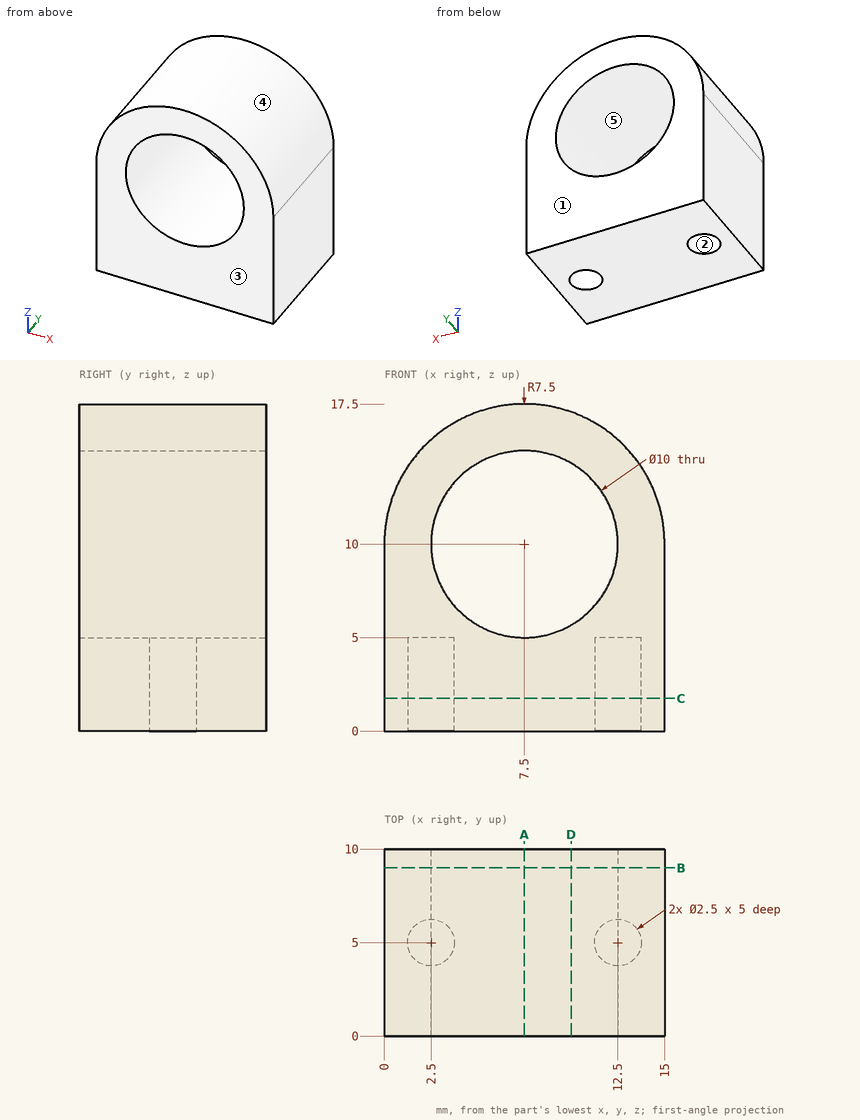
Could you check a few things on this drawing? It's one solid part, dimensions in mm from its lowest x, y, z. A direction names the side the tool comes from. Coordinates: 2 decimals unless noted, no trailing zeros. Loops run counter-clockwise (first coordinate to the right, second up) from the corner with the lowest first, then second, coordinate; pieces in that order, holes last. Notation, with made-up numbers: (4.25, -33) - (31.25, -33) arc R17 ccw to (31.25, -24) - close; hole circle Ø9 at (70.5, 68.25). An arc over 180 degrees is marked (long way). Answer as a JSON object with one key per item and string values. Group by question number.
Item 1: If we section it at A-A (x = 7.5): List the corners of the cut face in (y, z) for me, plus the area to 3 significant figures.
Item 2: If we section it at D-D (x = 10): List the corners of the cut face in (y, z) for me, plus the area to 3 significant figures.
Item 3: If I drill on L1, parallel to X at y = 5, z = 1.6; L2, parallel to Y at x = 12.5, z = 2.7; L3, parallel to Z at x = 10.25, y = 5.25, over which ranges is the centre line in solid material (lowest first)? Write a range as from..to.
Item 4: On a 3-axis mill with a long thin cutter (end or side, diameter ignored), from which of +Z, -Z, +X, -X, +Y, -Y can I reach the whole of each face in a straight line? I mean the marked faces 1 and 2. Say none if no direction works.
Item 5: If we section it at B-B (y = 9): List the corners of the cut face in (x, z) for me.
Item 6: If we mould it in two halves opening along Z, with no side actions, what happens to the marked faces 3, 4 and 5? For each: released by +Z, released by -Z, zero draft, split by the parting line, or undercut.
Item 7: For pin 1 (5 mm diameter, centred on x = 2.5, y = 4, fed in from +Z); pin 2 (0.8 mm diameter, centred on x = 12, y = 5.5, fed in from -Z); pin 3 (3 mm diameter, centred on x = 2.5, y = 5, fed in from +Z); pin 4 (3 mm diameter, centred on x = 5, z = 12, fed in from +Y), each with a flat end and sliding along its axis, tell me the tip position at first contact or that it passes through.
Item 8: If we section it at C-C (z = 1.75): List the corners of the cut face in (x, y) for me, plus the area to 3 significant figures.
Returned:
{
 "1": {"outline": "(0, 0) - (10, 0) - (10, 5) - (0, 5) - close; (0, 15) - (10, 15) - (10, 17.5) - (0, 17.5) - close", "area": "75.0 mm²"},
 "2": {"outline": "(0, 0) - (10, 0) - (10, 5.67) - (0, 5.67) - close; (0, 14.33) - (10, 14.33) - (10, 17.07) - (0, 17.07) - close", "area": "84.1 mm²"},
 "3": {"L1": "x = 0..1.25, 3.75..11.25, 13.75..15", "L2": "y = 0..3.75, 6.25..10", "L3": "z = 0..5.82, 14.18..16.98"},
 "4": {"face 1": "+Z, -Z, +X, -X, +Y", "face 2": "-Z"},
 "5": {"outline": "(0, 0) - (15, 0) - (15, 10) arc R7.5 ccw to (0, 10) - close; hole circle Ø10 at (7.5, 10)"},
 "6": {"face 3": "zero draft", "face 4": "released by +Z", "face 5": "undercut"},
 "7": {"pin 1": "stops at z = 17.07", "pin 2": "stops at z = 5", "pin 3": "stops at z = 16.63", "pin 4": "passes through"},
 "8": {"outline": "(0, 0) - (15, 0) - (15, 10) - (0, 10) - close; hole circle Ø2.5 at (2.5, 5); hole circle Ø2.5 at (12.5, 5)", "area": "140 mm²"}
}
